```python
from build123d import *

# Parameters (mm, degrees)
F1_DEPTH = 4
F2_R     = 3
F3_DEPTH = 20
F4_SIZE  = 1
F5_R     = 0.5


with BuildPart() as f1:
    # F0 (on Top) → F1 (new body)
    with BuildSketch(Plane.XY):
        Polygon((5, -2.886751), (5, 2.886751), (0, 5.773503), (-5, 2.886751), (-5, -2.886751), (0, -5.773503), align=None)
    extrude(amount=F1_DEPTH)

    # F2 (on face) → F3 (join)
    with BuildSketch(Plane.XY.offset(4)):
        Circle(F2_R)
    extrude(amount=F3_DEPTH)

    # F4
    f4_edges = [f1.edges().sort_by_distance(p)[0] for p in [
        (-3, 0, 24),
    ]]
    chamfer(f4_edges, length=F4_SIZE)

    # F5
    f5_edges = [f1.edges().sort_by_distance(p)[0] for p in [
        (0, -5.773503, 2),
        (5, -2.886751, 2),
        (5, 2.886751, 2),
        (-5, -2.886751, 2),
        (0, 5.773503, 2),
        (-5, 2.886751, 2),
    ]]
    fillet(f5_edges, radius=F5_R)


solid = f1.part
```
For this review, take the finished solid that the model builds, in its own axes (mm). A direction names the side the tool comes from. Give positions to 0.01 mm unless a question says otherwise; leave off trailing zeros. Write each loop counter-clockwise with the first axis right and the second up, starting at its lowest first coordinate (ties: lowest second). Pieces come first, ordered by that corner, then holes. Notation, with made-up numbers: M -40,76.5 L -33,76.5 A31 cw -33,105.5 Z; hole C 16.25,-18.75 d1. An arc over 180 degrees is marked long. Answer as CSV lines item,"result".
1. Consider section B-B, the plane y = 0. Write out the cut boundary in (x, z), then the cut area to 3 significant figures.
Findings:
outline,"M -5,0 L 5,0 L 5,4 L 3,4 L 3,23 L 2,24 L -2,24 L -3,23 L -3,4 L -5,4 Z"
area,"159 mm2"
2. For faces 1 (the flat face through (-2.469, 4.348, 1.972)), 2 (the cylindrical face through (-3, 0, 13)), list the 3-axis set-ups (+Z, -Z, +X, -X, +Y, -Y) from which the entire face can be reached by the end or side of a thin tool; tool diameter is ignored.
Findings:
face 1,"+Z, -Z, -X, +Y"
face 2,"+Z"
3. Wall thickness on line 1 (Z direction, x = 1.75, y = -3.25); line 2 (X direction, y = 0.25, z = 19.25); line 3 (Y direction, x = 0.75, z = 11): over which ranges is each line inside the solid? List them lowest first.
Findings:
line 1,"z = 0 to 4"
line 2,"x = -2.99 to 2.99"
line 3,"y = -2.9 to 2.9"
4. Consider section A-A, the plane x = 0. Write out the cut boundary in (y, z).
Findings:
outline,"M -5.7,0 L 5.7,0 L 5.7,4 L 3,4 L 3,23 L 2,24 L -2,24 L -3,23 L -3,4 L -5.7,4 Z"
5. For pin 1 (5 mm diameter, centred on y = 3.5, z = 18.5, fed in from +X); pin 2 (2 mm diameter, centred on y = 2.5, z = 13.5, fed in from -X); pin 3 (2 mm diameter, centred on x = 3, z = 7, fed in from -Y), all flat-tipped, find the tip position at first contact; note any pin that passes through.
Findings:
pin 1,"stops at x = 2.83"
pin 2,"stops at x = -2.6"
pin 3,"stops at y = -2.24"
6. Consider section C-C, the plane z = 7.5. Write out the cut boundary in (x, y), then the cut area to 3 significant figures.
Findings:
outline,"C 0,0 d6"
area,"28.3 mm2"
